Build history of the part. All positions in model axes, mm. A direction names the side the tool comes from. Round coordinates to 2 decimals unless told otherwise and drop trailing zeros. Order: outer loops, then holes, each group sorted by start corner. A loop starts at its lowest first (then second) coordinate and runs counter-clockwise, first axis right, second up. Notation, with made-up numbers: M 65,2.5 L 82,2.5 A22 ccw 82,17.5 Z; hole C -33,-6 d2. An arc over 180 degrees is marked long. One line per item, written item: value. Start each with the question number.
Item 1: Band-saw the part on B-B, the plane z = 4. Write the cut outline in (x, y), then the cut area to 3 significant figures.
Item 2: Band-saw the part on D-D, the plane x = 47.35. Write the cut outline in (y, z).
Item 3: Tool access for faces 4 (the flat face through (40.7, 10, 25)), 5 (the flat face through (3.8, 0.8, 0)): list every direction of +Z, -Z, +X, -X, +Y, -Y with a clear straight run to the whole face (end or side of a thin tool).
Item 4: Pin check, flat tips, straight feed: pin 1 (8 mm diameter, centred on x = -41, z = 44, fed in from +Y); pin 2 (15 mm diameter, centred on x = -3.5, z = 13, fed in from +Y). Stop position of each tip, or through.
Item 5: Band-saw the part on A-A, the plane y = 11. Write the cut outline in (x, z), then the cut area to 3 significant figures.
Item 6: Two-plate mould, pull along X, no slides. Class faces 1 (the flat face through (-55, 7, 25)), 2 (the flat face through (54, 10, 25)), 3 (the flat face through (55, 7, 25)): +X half, -X half, draft (parallel to the pull), parting line (faces both ways), or undercut.
Item 7: Probe L1, parallel to X at y = 7.5, z = 26; L2, parallel to X at y = 2.25, z = 14; L3, parallel to Y at x = 30.5, z = 28. List the from-to ranges inside material, lowest first.
Item 8: Band-saw the part on C-C, the plane y = 5.75. Write the cut outline in (x, z), then the cut area to 3 significant figures.
```python
from build123d import *

# Parameters (mm, degrees)
F2_DEPTH = 50
F3_R     = 1
F4_SIZE  = 0.5


with BuildPart() as f2:
    # F1 (on Top) → F2 (new body)
    with BuildSketch(Plane.XY):
        with BuildLine():
            Line((0, 1), (-39.7, 1))
            Line((-39.7, 1), (-39.7, 12.97))
            Line((-39.7, 12.97), (-40.7, 12.97))
            Line((-40.7, 12.97), (-40.7, 7.65))
            ThreePointArc((-40.7, 7.65), (-47.35, 1), (-54, 7.65))
            Line((-54, 7.65), (-54, 12.97))
            Line((-54, 12.97), (-55, 12.97))
            Line((-55, 12.97), (-55, 0))
            Line((-55, 0), (0, 0))
            Line((0, 0), (55, 0))
            Line((55, 0), (55, 12.97))
            Line((55, 12.97), (54, 12.97))
            Line((54, 12.97), (54, 7.65))
            ThreePointArc((54, 7.65), (47.35, 1), (40.7, 7.65))
            Line((40.7, 7.65), (40.7, 12.97))
            Line((40.7, 12.97), (39.7, 12.97))
            Line((39.7, 12.97), (39.7, 1))
            Line((39.7, 1), (0, 1))
        make_face()
    extrude(amount=F2_DEPTH)

    # F3
    f3_edges = [f2.edges().sort_by_distance(p)[0] for p in [
        (-55, 0, 25),
        (55, 0, 25),
        (39.7, 1, 25),
        (-39.7, 1, 25),
    ]]
    fillet(f3_edges, radius=F3_R)

    # F4
    f4_edges = [f2.edges().sort_by_distance(p)[0] for p in [
        (-54, 12.97, 25),
        (-40.7, 12.97, 25),
        (40.7, 12.97, 25),
        (54, 12.97, 25),
    ]]
    chamfer(f4_edges, length=F4_SIZE)


solid = f2.part
```
Output:
1. outline: M -55,1 A1 ccw -54,0 L 54,0 A1 ccw 55,1 L 55,12.97 L 54.5,12.97 L 54,12.47 L 54,7.65 A6.65 cw 40.7,7.65 L 40.7,12.47 L 40.2,12.97 L 39.7,12.97 L 39.7,2 A1 cw 38.7,1 L -38.7,1 A1 cw -39.7,2 L -39.7,12.97 L -40.2,12.97 L -40.7,12.47 L -40.7,7.65 A6.65 cw -54,7.65 L -54,12.47 L -54.5,12.97 L -55,12.97 Z
1. area: 195 mm²
2. outline: M 0,0 L 1,0 L 1,50 L 0,50 Z
3. face 4: +Z, -Z, +Y
3. face 5: -Z, +X, -X, +Y, -Y
4. pin 1: stops at y = 12.97
4. pin 2: stops at y = 1
5. outline: M -55,0 L -54,0 L -54,50 L -55,50 Z; M -40.7,0 L -39.7,0 L -39.7,50 L -40.7,50 Z; M 39.7,0 L 40.7,0 L 40.7,50 L 39.7,50 Z; M 54,0 L 55,0 L 55,50 L 54,50 Z
5. area: 200 mm²
6. face 1: -X half
6. face 2: undercut
6. face 3: +X half
7. L1: x = -55 to -54, -40.7 to -39.7, 39.7 to 40.7, 54 to 55
7. L2: x = -55 to -51.23, -43.47 to -39.7, 39.7 to 43.47, 51.23 to 55
7. L3: y = 0 to 1
8. outline: M -55,0 L -53.72,0 L -53.72,50 L -55,50 Z; M -40.98,0 L -39.7,0 L -39.7,50 L -40.98,50 Z; M 39.7,0 L 40.98,0 L 40.98,50 L 39.7,50 Z; M 53.72,0 L 55,0 L 55,50 L 53.72,50 Z
8. area: 255 mm²
